Job drawing, mm, ordinate dimensions from the low corner. One solid piece. A direction names the side the tool comes from. Give positions to 0.01 mm unless a question says otherwise; leave off trailing zeros. Write each loop counter-clockwise with the first axis right and the second up, starting at its lowest first coordinate (ties: lowest second). Pieces come first, ordered by that corner, then holes. Notation, with made-up numbers: (-9, 54.25) - (-3, 54.25) arc R27 ccw to (-3, 73.25) - close; hole circle Ø1 at (-37.5, 86.5). An arc over 180 degrees is marked (long way). Answer in a Markdown table with one row per item. Add a question column.
1. Band-saw the part on B-B on y = 99. Write the cut outline in (x, z), plus the area to 3 significant figures.
2. Band-saw the part on A-A on z = 9.25. Write the cut outline in (x, y) (1 decimal).
3. Which spindle directions (+Z, -Z, +X, -X, +Y, -Y) get a long thin tool onto all of the face, cutting with end or side? Do the marked faces 1 and 2. Say none if no direction does.
4. Drop flat-ended pins along their axis: pin 1 Ø3 at (y, z) = (58, 10.5) entering from -X (1 decimal); pin 2 Ø5 at (y, z) = (16.5, 7.5) entering from +X (1 decimal); pin 3 Ø1.5 at (y, z) = (15, 6.5) entering from +X (1 decimal). Give the stop position or say it passes through.
5. Probe line 1 along X through (y, z) = (87.5, 6.25); line 2 along Z through (x, y) = (21, 83.5); line 3 along Y through (x, z) = (12, 7.5) (1 decimal). List the from-to ranges inside material, lowest first.
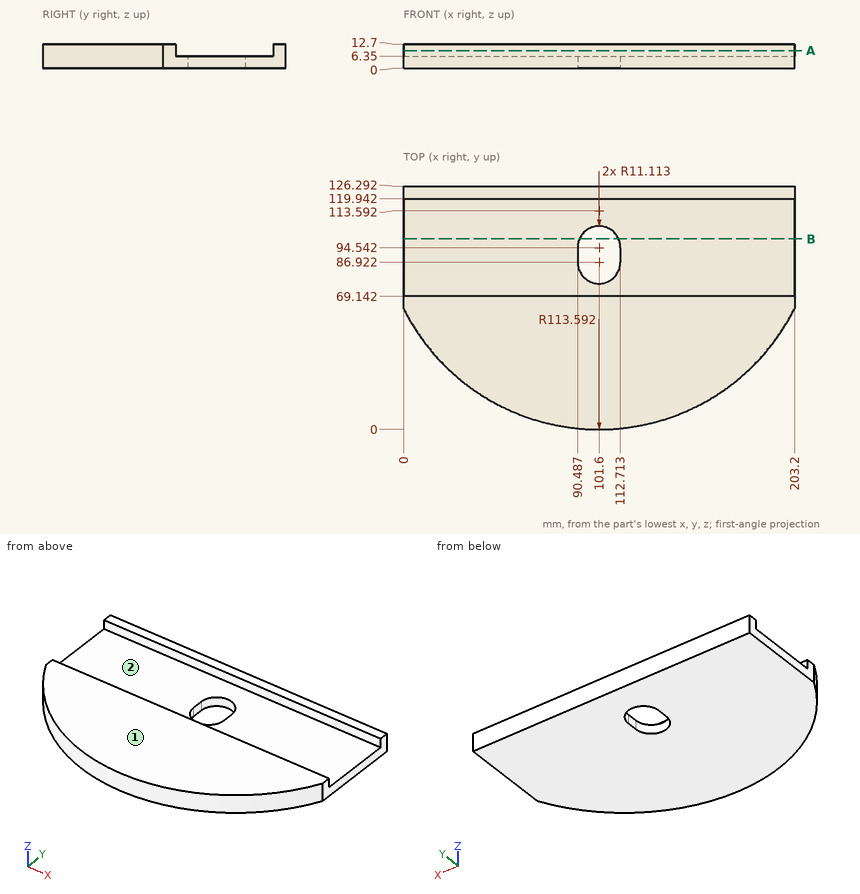
Values:
| question | item | result |
|---|---|---|
| 1 | outline | (0, 0) - (91.42, 0) - (91.42, 6.35) - (0, 6.35) - close; (111.78, 0) - (203.2, 0) - (203.2, 6.35) - (111.78, 6.35) - close |
| 1 | area | 1,160 mm² |
| 2 | outline | (0, 62.8) arc R113.6 ccw to (203.2, 62.8) - (203.2, 69.1) - (0, 69.1) - close; (0, 119.9) - (203.2, 119.9) - (203.2, 126.3) - (0, 126.3) - close |
| 3 | face 1 | +Z, +X, -X, +Y, -Y |
| 3 | face 2 | +Z, +X, -X |
| 4 | pin 1 | stops at x = 1.7 |
| 4 | pin 2 | stops at x = 164.5 |
| 4 | pin 3 | stops at x = 159.3 |
| 5 | line 1 | x = 0 to 90.49, 112.71 to 203.2 |
| 5 | line 2 | z = 0 to 6.35 |
| 5 | line 3 | y = 43.8 to 69.1, 119.9 to 126.3 |
